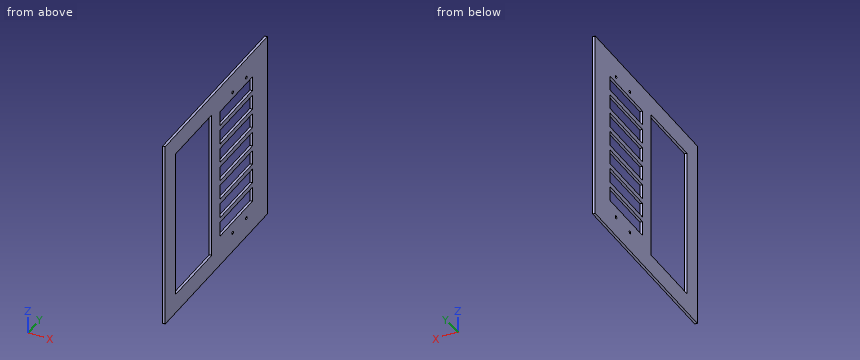
```python
from build123d import *

# Parameters (mm, degrees)
SKETCH001_W         = 501.65
SKETCH001_H         = 488.95
SKETCH001_R         = 3.81
SKETCH001_W_2       = 177.8
SKETCH001_H_2       = 387.35
PAD007_DEPTH        = 6.35
SKETCH005_W         = 158.75
SKETCH005_H         = 38.1
POCKET_DEPTH        = 6.35
LINEARPATTERN_COUNT = 7
LINEARPATTERN_PITCH = 50.8


with BuildPart() as part:
    # Sketch001 → Pad007 (new body)
    with BuildSketch(Plane(origin=(914.4, 1422.4, 914.4), x_dir=(0, 1, 0), z_dir=(-1, 0, 0))):
        Rectangle(SKETCH001_W, SKETCH001_H)
        with Locations((80.16875, 193.675)):
            Circle(SKETCH001_R, mode=Mode.SUBTRACT)
        with Locations((148.43125, 193.675)):
            Circle(SKETCH001_R, mode=Mode.SUBTRACT)
        with Locations((80.16875, -193.675)):
            Circle(SKETCH001_R, mode=Mode.SUBTRACT)
        with Locations((148.43125, -193.675)):
            Circle(SKETCH001_R, mode=Mode.SUBTRACT)
        with Locations((-111.125, 0)):
            Rectangle(SKETCH001_W_2, SKETCH001_H_2, mode=Mode.SUBTRACT)
    extrude(amount=PAD007_DEPTH)

    # Sketch005 → Pocket (cut)
    with BuildSketch(Plane(origin=(914.4, 1422.4, 914.4), x_dir=(0, 1, 0), z_dir=(1, 0, 0))):
        with Locations((98.425, 158.75)):
            Rectangle(SKETCH005_W, SKETCH005_H)
    pocket = extrude(amount=-POCKET_DEPTH, mode=Mode.SUBTRACT)

    # LinearPattern: Pocket ×7
    with Locations(*[(0, 0, -i * LINEARPATTERN_PITCH) for i in range(1, LINEARPATTERN_COUNT)]):
        add(pocket, mode=Mode.SUBTRACT)


solid = part.part
```
Model file for the job. Use its own axes, mm. Coordinates: 2 decimals unless noted, no trailing zeros. Order: outer loops, then holes, each group sorted by start corner. A loop starts at its lowest first (then second) coordinate and runs counter-clockwise, first axis right, second up. Notation, with made-up numbers: M 83.25,-10.5 L 107.25,-10.5 A27 ccw 107.25,9.5 Z; hole C 64.5,16 d1. An arc over 180 degrees is marked long. Answer as CSV lines item,"result".
(1) Wall check: line 1 along Y through (x, z) = (913.25, 815.5) (3 decimals); line 2 along Y through (x, z) = (914.25, 720.5) (3 decimals); line 3 along Y through (x, z) = (909.25, 789.5) (3 decimals). Give the ranges that are in metal, low to high.
Geometry says:
line 1,"y = 1171.575 to 1222.375, 1400.175 to 1441.45, 1600.2 to 1673.225"
line 2,"y = 1171.575 to 1498.765, 1506.372 to 1567.028, 1574.635 to 1673.225"
line 3,"y = 1171.575 to 1222.375, 1400.175 to 1673.225"
(2) Band-saw the part on B-B, the plane y = 1581.5. State how many separate pieces and enclosed holes the cut face has, then the cut area to 3 significant figures.
Geometry says:
separate pieces,"8"
enclosed holes,"0"
area,"1,410 mm2"
(3) Band-saw the part on C-C, the plane y = 1372.5. List the corners of the cut face in (x, z) (3 decimals).
Geometry says:
outline,"M 908.05,669.925 L 914.4,669.925 L 914.4,720.725 L 908.05,720.725 Z; M 908.05,1108.075 L 914.4,1108.075 L 914.4,1158.875 L 908.05,1158.875 Z"
(4) Band-saw the part on A-A, the plane z = 971. List the corners of the cut face in (x, y) (3 decimals).
Geometry says:
outline,"M 908.05,1171.575 L 914.4,1171.575 L 914.4,1222.375 L 908.05,1222.375 Z; M 908.05,1400.175 L 914.4,1400.175 L 914.4,1441.45 L 908.05,1441.45 Z; M 908.05,1600.2 L 914.4,1600.2 L 914.4,1673.225 L 908.05,1673.225 Z"
(5) Flat gauge pins, fed straight in: pin 1 (4.5 mm diameter, centred on y = 1502.57, z = 1108.08, fed in from -X); pin 2 (9 mm diameter, centred on y = 1570.83, z = 1108.08, fed in from +X). Where does each tip first touch, or does it go through?
Geometry says:
pin 1,"passes through"
pin 2,"stops at x = 914.4"
